```python
from build123d import *

# Parameters (mm, degrees)
SKETCH1_W           = 53.975
SKETCH1_H           = 88.9
SKETCH1_R           = 7.9375
SKETCH1_R_2         = 17.4625
BOSS_EXTRUDE1_DEPTH = 50.8
SKETCH5_R           = 2.09
CUT_EXTRUDE1_DEPTH  = 116.746060948
SKETCH5_3_R         = 3.6
CUT_EXTRUDE2_DEPTH  = 4.064
CUT_EXTRUDE3_DEPTH  = 2.54
FILLET1_R           = 1.27


with BuildPart() as part:
    # Sketch1 → Boss-Extrude1 (new body)
    with BuildSketch(Plane(origin=(0, 0, 0), x_dir=(0, 0, -1), z_dir=(1, 0, 0))):
        with Locations((26.9875, 44.45)):
            Rectangle(SKETCH1_W, SKETCH1_H)
        with Locations(Location((26.9875, 19.685, 0), (0, 0, 180))):
            Circle(SKETCH1_R, mode=Mode.SUBTRACT)
        with Locations(Location((26.9875, 60.325, 0), (0, 0, 180))):
            Circle(SKETCH1_R_2, mode=Mode.SUBTRACT)
    extrude(amount=BOSS_EXTRUDE1_DEPTH)

    # Sketch5 → Cut-Extrude1 (cut, through all)
    with BuildSketch(Plane.XY):
        with Locations((12.7, 83.34375)):
            Circle(SKETCH5_R)
        with Locations((12.7, 35.2425)):
            Circle(SKETCH5_R)
        with Locations((38.1, 83.34375)):
            Circle(SKETCH5_R)
        with Locations((38.1, 35.2425)):
            Circle(SKETCH5_R)
        with Locations((12.7, 5.87375)):
            Circle(SKETCH5_R)
        with Locations((38.1, 5.87375)):
            Circle(SKETCH5_R)
    extrude(amount=-CUT_EXTRUDE1_DEPTH, mode=Mode.SUBTRACT)

    # Sketch5<3> → Cut-Extrude2 (cut)
    with BuildSketch(Plane.XY):
        with Locations((38.1, 35.2425)):
            Circle(SKETCH5_3_R)
        with Locations((12.7, 83.34375)):
            Circle(SKETCH5_3_R)
        with Locations((38.1, 83.34375)):
            Circle(SKETCH5_3_R)
        with Locations((12.7, 35.2425)):
            Circle(SKETCH5_3_R)
        with Locations((38.1, 5.87375)):
            Circle(SKETCH5_3_R)
        with Locations((12.7, 5.87375)):
            Circle(SKETCH5_3_R)
    extrude(amount=-CUT_EXTRUDE2_DEPTH, mode=Mode.SUBTRACT)

    # Sketch6 → Cut-Extrude3 (cut)
    with BuildSketch(Plane(origin=(0, 0, -53.975), x_dir=(-1, 0, 0), z_dir=(0, 0, -1))):
        Polygon((-34.02855, 83.34375), (-36.064275, 86.86972913), (-40.135725, 86.86972913), (-42.17145, 83.34375), (-40.135725, 79.81777087), (-36.064275, 79.81777087), align=None)
        Polygon((-8.62855, 83.34375), (-10.664275, 86.86972913), (-14.735725, 86.86972913), (-16.77145, 83.34375), (-14.735725, 79.81777087), (-10.664275, 79.81777087), align=None)
        Polygon((-8.62855, 35.2425), (-10.664275, 38.76847913), (-14.735725, 38.76847913), (-16.77145, 35.2425), (-14.735725, 31.71652087), (-10.664275, 31.71652087), align=None)
        Polygon((-34.02855, 35.2425), (-36.064275, 38.76847913), (-40.135725, 38.76847913), (-42.17145, 35.2425), (-40.135725, 31.71652087), (-36.064275, 31.71652087), align=None)
        Polygon((-34.02855, 5.87375), (-36.064275, 9.39972913), (-40.135725, 9.39972913), (-42.17145, 5.87375), (-40.135725, 2.34777087), (-36.064275, 2.34777087), align=None)
        Polygon((-8.62855, 5.87375), (-10.664275, 9.39972913), (-14.735725, 9.39972913), (-16.77145, 5.87375), (-14.735725, 2.34777087), (-10.664275, 2.34777087), align=None)
    extrude(amount=-CUT_EXTRUDE3_DEPTH, mode=Mode.SUBTRACT)

    # Fillet1
    fillet1_edges = [part.edges().sort_by_distance(p)[0] for p in [
        (0, 60.325, -44.45),
        (50.8, 60.325, -44.45),
        (50.8, 88.9, -26.9875),
        (0, 19.685, -34.925),
        (50.8, 19.685, -34.925),
        (50.8, 44.45, 0),
        (50.8, 0, -26.9875),
        (0, 44.45, 0),
        (0, 88.9, -26.9875),
        (0, 44.45, -53.975),
        (0, 0, -26.9875),
        (25.4, 0, 0),
        (25.4, 88.9, 0),
        (25.4, 88.9, -53.975),
        (25.4, 0, -53.975),
        (50.8, 44.45, -53.975),
    ]]
    fillet(fillet1_edges, radius=FILLET1_R)

    # SurfaceCut1
    split(bisect_by=Plane.XY.offset(-26.9875), keep=Keep.BOTTOM)


solid = part.part
```
Here's how the part is built. I have some questions about the finished solid (model axes, mm). A direction names the side the tool comes from. Give positions to 0.01 mm unless a question says otherwise; leave off trailing zeros. Loops run counter-clockwise (first coordinate to the right, second up) from the corner with the lowest first, then second, coordinate; pieces in that order, holes last. Notation, with made-up numbers: M 87,41.25 L 106,41.25 A20 ccw 106,45.25 Z; hole C -28.5,77 d1. An arc over 180 degrees is marked long. Use one line per item in the form item = value. Start each with the question number.
Q1. If we section it at B-B (z = -49): Write out the boundary of the cut face in (x, y), then the cut area to 3 significant figures.
Q2. Which directions (+Z, -Z, +X, -X, +Y, -Y) give clear straight access to the entire face, cutting with the end or side of a thin tool? Please do faces 4 (the flat face through (36, 7, -51.435)), 5 (the cylindrical face through (13.824, 37.005, -39.04)).
Q3. If we section it at A-A (x = 38.1): State how many separate pieces and enclosed holes the cut face has, then the cut area to 3 significant figures.
Q4. I need wall thicknesses on line 1 along Y through (x, z) = (12.7, -46.25); line 2 along X through (y, z) = (82, -28.75); line 3 along Y through (x, z) = (42, -31.5). Which ranges of each line are inside material? Lowest first, please.
Q5. Will these pins go through, and if not, where does the flat tip stop? pin 1 Ø5 at (y, z) = (43.5, -39) entering from -X; pin 2 Ø8 at (x, y) = (32.5, 19) entering from +Z; pin 3 Ø3.5 at (x, y) = (12.7, 5.87) entering from -Z; pin 4 Ø5.5 at (x, y) = (12.7, 83.34) entering from -Z (3 decimals).
Q6. Thinking about a two-plate mould opening in Y: for faces 1 (the flat face through (25, 6, -26.988)), 2 (the flat face through (35.03, 85.08, -52.72)), 3 (the flat face through (35.03, 7.61, -52.72)), which applies, +Y half, -Y half, draft (parallel to the pull), parting line (faces both ways), or undercut?
Taken from the geometry:
q1.outline = M 0,1.27 A1.27 ccw 1.27,0 L 49.53,0 A1.27 ccw 50.8,1.27 L 50.8,87.63 A1.27 ccw 49.53,88.9 L 1.27,88.9 A1.27 ccw 0,87.63 Z; hole C 12.7,5.87 d4.18; hole C 12.7,35.24 d4.18; hole C 12.7,83.34 d4.18; hole C 38.1,5.87 d4.18; hole C 38.1,35.24 d4.18; hole C 38.1,83.34 d4.18
q1.area = 4,430 mm^2
q2.face_4 = -Z
q2.face_5 = +Z, -Z
q3.separate_pieces = 4
q3.enclosed_holes = 0
q3.area = 1,460 mm^2
q4.line_1 = 0 to 3.78, 7.96 to 33.15, 37.33 to 81.25, 85.43 to 88.9
q4.line_2 = 0 to 11.1, 14.3 to 36.5, 39.7 to 50.8
q4.line_3 = 0 to 13.15, 26.22 to 43.46, 77.19 to 88.9
q5.pin_1 = 0
q5.pin_2 = -33.39
q5.pin_3 = through
q5.pin_4 = -51.435
q6.face_1 = draft
q6.face_2 = undercut
q6.face_3 = undercut
